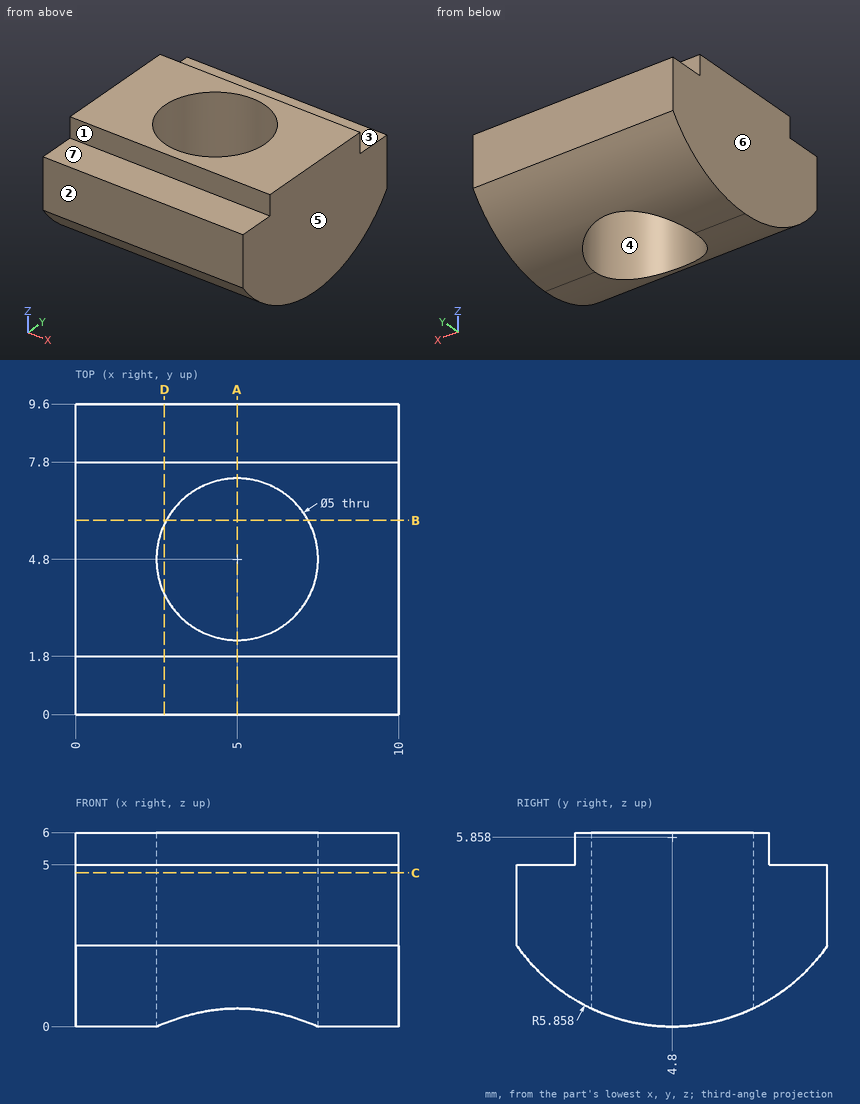
Study the drawing (mm; zero at the part's minimum x, y, z) and answer. A direction names the side the tool comes from. Round coordinates to 2 decimals unless told otherwise and drop trailing zeros. Order: outer loops, then holes, each group sorted by start corner. A loop starts at its lowest first (then second) coordinate and runs counter-clockwise, first axis right, second up. Notation, with made-up numbers: M -19.75,-2.5 L 20.25,-2.5 A17 cw 20.25,2.5 Z; hole C 37,62.25 d11. An arc over 180 degrees is marked long. One line per item, written item: value.
Q1. For the marked faces 1, 2 and 3, determine the directions among +Z, -Z, +X, -X, +Y, -Y from which every point of the face is accessible in a straight line to the end or side of a thin tool.
Derived:
face 1: +Z, +X, -X, -Y
face 2: +Z, -Z, +X, -X, -Y
face 3: +Z, +X, -X, +Y
Q2. Straight lines are drawn through the part: line 1 (Y direction, x = 5, z = 4.75); line 2 (Y direction, x = 3.5, z = 1); line 3 (Y direction, x = 1, z = 5.5). For each, find the intervals that lie inside material, in ascending order.
Derived:
line 1: 0 to 2.3, 7.3 to 9.6
line 2: 1.53 to 2.8, 6.8 to 8.07
line 3: 1.8 to 7.8
Q3. Flat-ended cylindrical pins translate along their axes: pin 1 (0.5 mm diameter, centred on x = 6, y = 8.5, fed in from +Z); pin 2 (5 mm diameter, centred on x = 5, y = 8.5, fed in from -Z); pin 3 (1.5 mm diameter, centred on x = 6.5, z = 1, fed in from -Y). Find the tip coordinate at first contact, or state that the pin passes through.
Derived:
pin 1: z = 5
pin 2: z = 0.3
pin 3: y = 0.62
Q4. Find section C-C on z = 4.75. Write down the section's boundary in (x, y).
Derived:
outline: M 0,0 L 10,0 L 10,9.6 L 0,9.6 Z; hole C 5,4.8 d5
Q5. Find section A-A on x = 5. Write down the section's boundary in (y, z), then the cut area to 3 significant figures.
Derived:
outline: M 0,2.5 A5.86 ccw 2.3,0.56 L 2.3,6 L 1.8,6 L 1.8,5 L 0,5 Z; M 7.3,0.56 A5.86 ccw 9.6,2.5 L 9.6,5 L 7.8,5 L 7.8,6 L 7.3,6 Z
area: 17.8 mm²
Q6. Find section B-B on y = 6. Write down the section's boundary in (x, z).
Derived:
outline: M 0,0.12 L 2.81,0.12 L 2.81,6 L 0,6 Z; M 7.19,0.12 L 10,0.12 L 10,6 L 7.19,6 Z
Q7. Find section D-D on x = 2.75. Write down the section's boundary in (y, z).
Derived:
outline: M 0,2.5 A5.86 ccw 3.71,0.1 L 3.71,6 L 1.8,6 L 1.8,5 L 0,5 Z; M 5.89,0.1 A5.86 ccw 9.6,2.5 L 9.6,5 L 7.8,5 L 7.8,6 L 5.89,6 Z
Q8. Determine the mould class of the marked faces 4, 5, 6 and 7 for opening direction X: released by +X, released by -X, zero draft, split by the parting line, or undercut.
Derived:
face 4: undercut
face 5: released by +X
face 6: released by -X
face 7: zero draft
